from build123d import *

# Parameters (mm, degrees)
SKETCH_W     = 62
SKETCH_H     = 50
PAD_DEPTH    = 3.75
SKETCH001_W  = 1.25
SKETCH001_H  = 23
PAD001_DEPTH = 3


with BuildPart() as part:
    # Sketch → Pad (new body, symmetric)
    with BuildSketch(Plane.XY):
        with Locations((31, 25)):
            Rectangle(SKETCH_W, SKETCH_H)
    extrude(amount=PAD_DEPTH, both=True)

    # Sketch001 → Pad001 (join, symmetric)
    with BuildSketch(Plane.XY):
        with Locations((-0.625, 11.5)):
            Rectangle(SKETCH001_W, SKETCH001_H)
    extrude(amount=PAD001_DEPTH, both=True)


solid = part.part
Build history of the part. All positions in model axes, mm. A direction names the side the tool comes from. Round coordinates to 2 decimals unless told otherwise and drop trailing zeros. Loops run counter-clockwise (first coordinate to the right, second up) from the corner with the lowest first, then second, coordinate; pieces in that order, holes last. Notation, with made-up numbers: (-1, 44) -> (48, 44) arc R16 ccw to (48, 54) -> close; hole circle Ø10 at (5, -15.5). An arc over 180 degrees is marked (long way). Use CSV: the item, a comma, the result in double quotes. Start each with the question number.
Q1. Flat gauge pins, fed straight in: pin 1 Ø2 at (y, z) = (26, 1.5) entering from -X; pin 2 Ø0.6 at (x, y) = (-0.5, 13.5) entering from +Z; pin 3 Ø0.6 at (x, z) = (-0.5, 0) entering from +Y. Where does each tip first touch, or does it go through?
Q2. Mould opens along Y. For faces 1 (the face through (-1, 23, 0)), 2 (the face through (31, 25, 3.75)), 3 (the face through (30, 0, 0)) say: +Y half, -Y half, draft (parallel to the pull), parting line (faces both ways), or undercut.
Q3. Drill centre line: L1, parallel to X at y = 25, z = -0.5. Where is it in solid material? Low to high.
Q4. Saw through at A-A on y = 26. Give the cut face in (x, z), and give its area (3 significant figures).
Q5. Which spindle directions (+Z, -Z, +X, -X, +Y, -Y) get a long thin tool onto all of the face, cutting with end or side? Do faces 4 (the face through (31, 50, 0)), 5 (the face through (-1, 12, 3)), 6 (the face through (-1, 12, -3)). Say none if no direction does.
Solutions:
1,pin 1,"stops at x = 0"
1,pin 2,"stops at z = 3"
1,pin 3,"stops at y = 23"
2,face 1,"+Y half"
2,face 2,"draft"
2,face 3,"-Y half"
3,L1,"x = 0 to 62"
4,outline,"(0, -3.75) -> (62, -3.75) -> (62, 3.75) -> (0, 3.75) -> close"
4,area,"465 mm^2"
5,face 4,"+Z, -Z, +X, -X, +Y"
5,face 5,"+Z, -X, +Y, -Y"
5,face 6,"-Z, -X, +Y, -Y"
